```python
from build123d import *

# Parameters (mm, degrees)
F2_SIZE = 1


with BuildPart() as f1:
    # F0 (on Front) → F1 (revolve)
    with BuildSketch(Plane.XZ):
        Polygon((0, 4), (0, 0), (55.8, 0), (55.8, 4), (53.8, 4), (53.8, 3), (52.9, 3), (52.9, 4), (2.9, 4), (2.9, 3), (2, 3), (2, 4), align=None)
    revolve(axis=Axis((27.761492, 0, 0), (1, 0, 0)))

    # F2
    f2_edges = [f1.edges().sort_by_distance(p)[0] for p in [
        (55.8, 0, -4),
        (0, 0, -4),
    ]]
    chamfer(f2_edges, length=F2_SIZE)


solid = f1.part
```
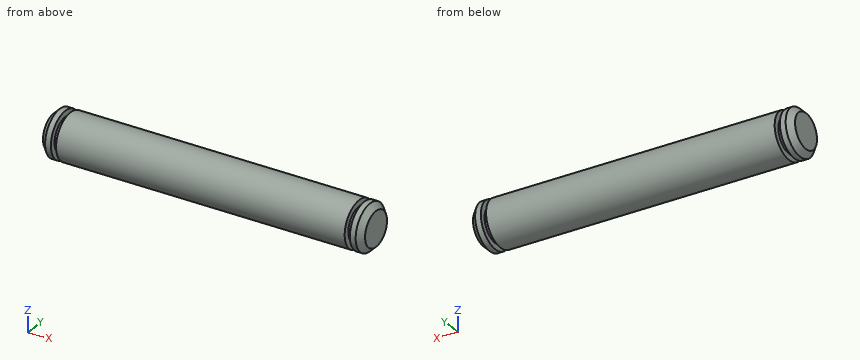
Check sheet for the modelled part. Datum: model origin and axes. Units: mm. Give positions to 0.01 mm unless a question says otherwise; leave off trailing zeros. Loops run counter-clockwise (first coordinate to the right, second up) from the corner with the lowest first, then second, coordinate; pieces in that order, holes last. Notation, with made-up numbers: (82, 66) - (128, 66) arc R28 cw to (128, 94) - close; hole circle Ø1 at (-0.5, 1.5). An arc over 180 degrees is marked (long way). One line per question, with ' | ' between items. Start each with the question number.
1. Cross-section at A-A, the plane x = 29. Enter the section's corners in (y, z).
2. Gauge pin test, flat ends, axial feed: pin 1 Ø2 at (y, z) = (-1, -1) entering from -X; pin 2 Ø3 at (x, y) = (29, -2.5) entering from +Z; pin 3 Ø2 at (x, y) = (36.5, -3) entering from -Z. Record the tip position at first contact, or that the pin passes through.
3. Material ranges on line 1 along X through (y, z) = (-2, 3.25); line 2 along X through (y, z) = (0.5, 3.5); line 3 along Y through (x, z) = (37, -1.5), recorded low to high. Write a range as [from, to].
Check result:
1) outline: circle Ø8 at (0, 0)
2) pin 1: stops at x = 0 | pin 2: stops at z = 3.87 | pin 3: stops at z = -3.46
3) line 1: x = [0.82, 2], [2.9, 52.9], [53.8, 54.98] | line 2: x = [0.54, 2], [2.9, 52.9], [53.8, 55.26] | line 3: y = [-3.71, 3.71]
